The listing builds one solid part. Answer for the finished solid, in the listing's coordinates (mm). Face numbers are marked on the shaded views. A direction names the side the tool comes from. Coordinates: 2 decimals unless noted, no trailing zeros. Loops run counter-clockwise (first coordinate to the right, second up) from the corner with the lowest first, then second, coordinate; pieces in that order, holes last. Notation, with made-up numbers: M 0,-38 L 37,-38 A21 ccw 37,-12 Z; hole C -1,-16 d4. An arc over 180 degrees is marked long. Return JSON: item names as keys, results as strings. Group by question number.
1. Section A-A (z = 0) is taken. Write down the section's boundary in (x, y).
2. Straight lines are drawn through the part: L1, parallel to Y at x = 0, z = -0.75; L2, parallel to Y at x = -56, z = 22.5; L3, parallel to Z at x = 3, y = 66.5. For each, find the intervals that lie inside material, in ascending order. Write a range as from..to.
3. The mould has two halves that part along Y. Classify the marked faces 3, 4 and 5: pulls with the +Y half, pulls with the -Y half, needs draft (parallel to the pull), parting line crosses it, or undercut.
4. Which of the six approach directions +Z, -Z, +X, -X, +Y, -Y give full straight-line access (tool end or side, diameter ignored) to the marked faces 1 and 2?
5. Given P1, Ø16, axis at x = 0, y = 100, coming from the -Z side; P2, Ø12, axis at x = 0, y = 102.5, coming from the +Z side; P3, Ø12, axis at y = 22.5, z = 35, coming from the +X side, each flat-ended and moving along its own axis, determine where each tip first touches the part or whether it passes through.
```python
from build123d import *

# Parameters (mm, degrees)
SKETCH1_R           = 75
BOSS_EXTRUDE1_DEPTH = 20
FILLET1_R           = 5
BOSS_EXTRUDE2_DEPTH = 5
CHAMFER1_SIZE       = 2.5
FILLET2_R           = 5
SKETCH3_R           = 10
BOSS_EXTRUDE3_DEPTH = 5
CHAMFER2_SIZE       = 2.5
SKETCH4_R           = 5
CUT_EXTRUDE1_DEPTH  = 10


with BuildPart() as part:
    # Sketch1 → Boss-Extrude1 (new body)
    with BuildSketch(Plane(origin=(0, 0, 0), x_dir=(1, 0, 0), z_dir=(0, 1, 0))):
        Circle(SKETCH1_R)
    extrude(amount=BOSS_EXTRUDE1_DEPTH)

    # Fillet1
    fillet1_edges = [part.edges().sort_by_distance(p)[0] for p in [
        (-75, 20, 0),
    ]]
    fillet(fillet1_edges, radius=FILLET1_R)

    # Sketch2 → Boss-Extrude2 (add, symmetric)
    with BuildSketch(Plane.XY):
        with BuildLine():
            Line((-35, 15), (30, 15))
            ThreePointArc((30, 15), (17.428098582, 56.126843631), (14.970645506, 99.06203778))
            ThreePointArc((14.970645506, 99.06203778), (6.012327577, 113.742340307), (-10.849201429, 110.358321696))
            ThreePointArc((-10.849201429, 110.358321696), (-35.460543036, 65.854059614), (-35, 15))
        make_face()
    extrude(amount=BOSS_EXTRUDE2_DEPTH, both=True)

    # Chamfer1
    chamfer1_edges = [part.edges().sort_by_distance(p)[0] for p in [
        (16.970295051, 58.803839559, -5),
        (6.012327577, 113.742340307, -5),
        (-34.796467261, 68.341174934, -5),
        (16.970295051, 58.803839559, 5),
        (6.012327577, 113.742340307, 5),
        (-34.796467261, 68.341174934, 5),
    ]]
    chamfer(chamfer1_edges, length=CHAMFER1_SIZE)

    # Fillet2
    fillet2_edges = [part.edges().sort_by_distance(p)[0] for p in [
        (-4.241511046, 20, -5),
        (-4.241511046, 20, 5),
    ]]
    fillet(fillet2_edges, radius=FILLET2_R)

    # Sketch3 → Boss-Extrude3 (add)
    with BuildSketch(Plane.XY.offset(5)):
        with Locations((0, 100)):
            Circle(SKETCH3_R)
    extrude(amount=BOSS_EXTRUDE3_DEPTH)

    # Chamfer2
    chamfer2_edges = [part.edges().sort_by_distance(p)[0] for p in [
        (-10, 100, 10),
    ]]
    chamfer(chamfer2_edges, length=CHAMFER2_SIZE)

    # Sketch4 → Cut-Extrude1 (cut)
    with BuildSketch(Plane(origin=(0, 0, -5), x_dir=(-1, 0, 0), z_dir=(0, 0, -1))):
        with Locations((0, 100)):
            Circle(SKETCH4_R)
    extrude(amount=-CUT_EXTRUDE1_DEPTH, mode=Mode.SUBTRACT)


solid = part.part
```
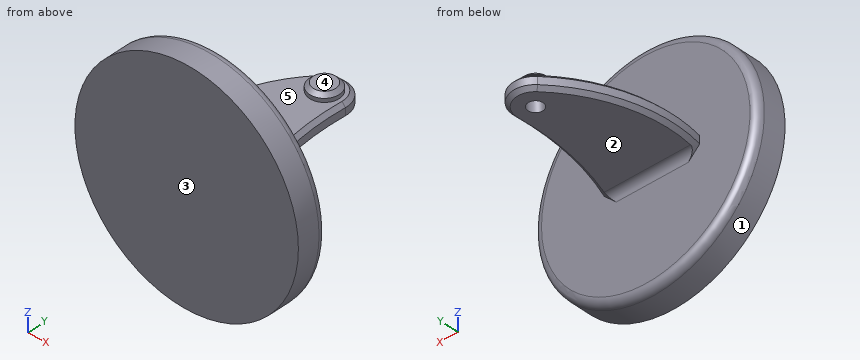
Worked out:
{
 "1": {"outline": "M -75,0 L 75,0 L 75,15 A5 ccw 70,20 L 27.88,20 A180 cw 14.97,99.06 A15 ccw -10.85,110.36 A100 ccw -36.23,20 L -70,20 A5 ccw -75,15 Z; hole C 0,100 d10"},
 "2": {"L1": "0..95, 105..115", "L2": "0..20", "L3": "-5..5"},
 "3": {"face 3": "pulls with the -Y half", "face 4": "needs draft", "face 5": "undercut"},
 "4": {"face 1": "+Y, -Y", "face 2": "-Z, +X, -X, +Y"},
 "5": {"P1": "z = -5", "P2": "z = 10", "P3": "x = 67.24"}
}
